from build123d import *

# Parameters (mm, degrees)
SKETCH1_R           = 19.05
BOSS_EXTRUDE1_DEPTH = 25.4
SKETCH3_R           = 25.4
BOSS_EXTRUDE2_DEPTH = 25.4
SKETCH4_R           = 50.8
SKETCH4_R_2         = 25.4
BOSS_EXTRUDE3_DEPTH = 25.4
BOSS_EXTRUDE4_DEPTH = 101.6


with BuildPart() as part:
    # Sketch1 → Boss-Extrude1 (new body)
    with BuildSketch(Plane.XY):
        with BuildLine():
            Line((-78.509090909, 38.1), (99.290909091, 38.1))
            ThreePointArc((99.290909091, 38.1), (137.390909091, 0), (99.290909091, -38.1))
            Line((99.290909091, -38.1), (-78.509090909, -38.1))
            ThreePointArc((-78.509090909, -38.1), (-116.609090909, 0), (-78.509090909, 38.1))
        make_face()
        with Locations((-78.509090909, 0)):
            Circle(SKETCH1_R, mode=Mode.SUBTRACT)
        with Locations((99.290909091, 0)):
            Circle(SKETCH1_R, mode=Mode.SUBTRACT)
    extrude(amount=-BOSS_EXTRUDE1_DEPTH)



with BuildPart() as body_2:
    # Sketch3 → Boss-Extrude2 (new body)
    with BuildSketch(Plane(origin=(0, 0, -82.55), x_dir=(-1, 0, 0), z_dir=(0, 0, -1))):
        with BuildLine():
            Line((-61.190909091, 127), (-61.190909091, 38.1))
            Line((-61.190909091, 38.1), (40.409090909, 38.1))
            Line((40.409090909, 38.1), (40.409090909, 127))
            ThreePointArc((40.409090909, 127), (-10.390909091, 177.8), (-61.190909091, 127))
        make_face()
        with Locations((-10.390909091, 127)):
            Circle(SKETCH3_R, mode=Mode.SUBTRACT)
    extrude(amount=BOSS_EXTRUDE2_DEPTH)

    # Sketch4 → Boss-Extrude3 (add)
    with BuildSketch(Plane(origin=(0, 0, -107.95), x_dir=(-1, 0, 0), z_dir=(0, 0, -1))):
        with Locations((-10.390909091, 127)):
            Circle(SKETCH4_R)
        with Locations((-10.390909091, 127)):
            Circle(SKETCH4_R_2, mode=Mode.SUBTRACT)
    extrude(amount=BOSS_EXTRUDE3_DEPTH)


with BuildPart() as part_1:
    add(part.part)

    add(body_2.part)  # Boss-Extrude4 merges body 2
    # Sketch6 → Boss-Extrude4 (add)
    with BuildSketch(Plane(origin=(61.190909091, 0, 0), x_dir=(0, 0, -1), z_dir=(1, 0, 0))):
        with BuildLine():
            Line((25.4, 38.1), (66.869857518, 38.1))
            ThreePointArc((66.869857518, 38.1), (78.035050252, 40.707035383), (82.55, 51.246171546))
            Line((82.55, 51.246171546), (107.95, 51.246171546))
            ThreePointArc((107.95, 51.246171546), (99.806428385, 23.245891332), (74.248865658, 9.205078029))
            Line((74.248865658, 9.205078029), (25.4, 9.205078029))
            Line((25.4, 9.205078029), (25.4, 38.1))
        make_face()
    extrude(amount=-BOSS_EXTRUDE4_DEPTH)


solid = part_1.part
Input: part model. Units: mm. Frame: model coordinates. A direction names the side the tool comes from. Coordinates: 2 decimals unless noted, no trailing zeros. Loops run counter-clockwise (first coordinate to the right, second up) from the corner with the lowest first, then second, coordinate; pieces in that order, holes last.
(1) Section D-D on x = -4.5. Return the cut outline in (y, z), then the cut area to 3 significant figures.
(2) Material intervals for probe 1 along Y at (x, z) = (-20, -8); probe 2 along Z at (x, y) = (8.5, 152.5); probe 3 along Z at (x, y) = (7, 4), sorted ascending.
(3) Pull-direction query (Y, two-part tool) for faces 6 (the face through (12, 38.1, -26)), 7 (the face through (-0.2, 150.3, -133.35)), 8 (the face through (11.1, 47.13, -108.18)); classes: released by +Y, released by -Y, zero draft, split by the parting line, or undercut.
(4) Section B-B on z = -85.5. Return the cut outline in (x, y).
(5) Section A-A on y = 0. Return the cut outline in (x, z).
(6) Section C-C on y = 109.5. Return the cut outline in (x, z).
(7) Set-up query: faces 1 (the face through (11, 9.205, -50)), 2 (the face through (-40.409, 56, -86)), 3 (the face through (61.191, 56, -86)), 4 (the face through (11, 100, -82.55)), 5 (the face through (17, 177.37, -113.24)). Return all of +Z, -Z, +X, -X, +Y, -Y with unobstructed straight access to the full face (end or side cutting, diameter ignored); none if empty.
(8) First-contact query: pin 1 Ø20 at (x, z) = (44.5, -28.5) entering from +Y; pin 2 Ø6 at (y, z) = (65, -81.5) entering from +X; pin 3 Ø5 at (x, y) = (33.5, 70) entering from +Z. Flat tips, straight axial feed; report the tip coordinate or a pass-through.
Data:
1. outline: (-38.1, -25.4) - (9.21, -25.4) - (9.21, -74.25) arc R38.1 ccw to (38.1, -107.11) - (38.1, -107.95) - (42.91, -107.95) arc R38.1 ccw to (51.25, -107.95) - (78.43, -107.95) - (78.43, -133.35) - (106.42, -133.35) - (106.42, -82.55) - (49.63, -82.55) arc R12.7 cw to (38.1, -66.87) - (38.1, 0) - (-38.1, 0) - close; (147.58, -133.35) - (175.57, -133.35) - (175.57, -82.55) - (147.58, -82.55) - close
1. area: 7,930 mm2
2. probe 1: y = -38.1 to 38.1
2. probe 2: z = -133.35 to -82.55
2. probe 3: z = -25.4 to 0
3. face 6: released by +Y
3. face 7: zero draft
3. face 8: undercut
4. outline: (-40.41, 12.24) - (61.19, 12.24) - (61.19, 127) arc R50.8 ccw to (-40.41, 127) - close; hole circle Ø50.8 at (10.39, 127)
5. outline: (-116.61, -25.4) - (-97.56, -25.4) - (-97.56, 0) - (-116.61, 0) - close; (-59.46, -25.4) - (80.24, -25.4) - (80.24, 0) - (-59.46, 0) - close; (118.34, -25.4) - (137.39, -25.4) - (137.39, 0) - (118.34, 0) - close
6. outline: (-40.41, -107.95) - (-37.3, -107.95) - (-37.3, -133.35) - (-8.02, -133.35) - (-8.02, -82.55) - (-40.41, -82.55) - close; (28.8, -133.35) - (58.08, -133.35) - (58.08, -107.95) - (61.19, -107.95) - (61.19, -82.55) - (28.8, -82.55) - close
7. face 1: -Z, +X, -X, -Y
7. face 2: -Z, -X, +Y, -Y
7. face 3: -Z, +X, +Y, -Y
7. face 4: +Z, +X, -X, +Y
7. face 5: -Z
8. pin 1: stops at y = 38.1
8. pin 2: stops at x = 61.19
8. pin 3: stops at z = -82.55
